Work out the finished part from the listing and answer in its coordinate system (mm). Face numbers are marked on the shaded views. A direction names the side the tool comes from. Round coordinates to 2 decimals unless told otherwise and drop trailing zeros. Loops run counter-clockwise (first coordinate to the right, second up) from the corner with the lowest first, then second, coordinate; pieces in that order, holes last. Notation, with made-up numbers: M -36.5,46.25 L -28.5,46.25 A8 ccw -28.5,52.25 Z; hole C 17.5,7.5 d4. An arc over 180 degrees is marked long. One line per item, written item: value.
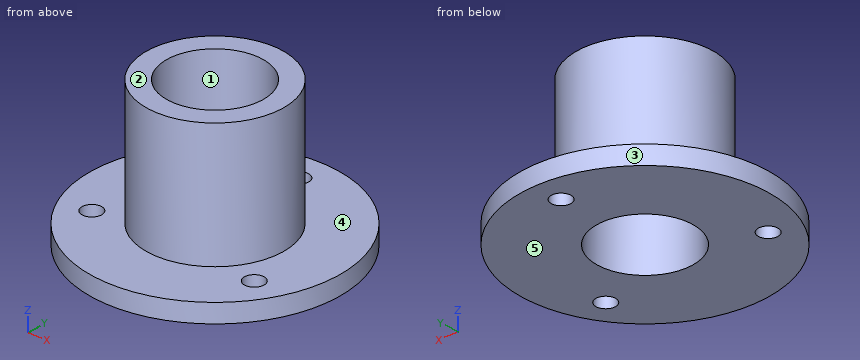
```python
from build123d import *

# Parameters (mm, degrees)
F0_R     = 11
F0_R_2   = 7.75
F1_DEPTH = 23
F0_R_3   = 20
F0_R_4   = 1.5875
F2_DEPTH = 3


with BuildPart() as f1:
    # F0 (on Top) → F1 (new body)
    with BuildSketch(Plane.XY):
        Circle(F0_R)
        Circle(F0_R_2, mode=Mode.SUBTRACT)
    extrude(amount=F1_DEPTH)

    # F0 (on Top) → F2 (join)
    with BuildSketch(Plane.XY):
        Circle(F0_R_3)
        with Locations((-13.282665, -7.66875)):
            Circle(F0_R_4, mode=Mode.SUBTRACT)
        with Locations((13.282665, -7.66875)):
            Circle(F0_R_4, mode=Mode.SUBTRACT)
        Circle(F0_R, mode=Mode.SUBTRACT)
        with Locations((0, 15.3375)):
            Circle(F0_R_4, mode=Mode.SUBTRACT)
    extrude(amount=F2_DEPTH)


solid = f1.part
```
1) Find section B-B (y = 0). Give the vertices of the cut face in (x, z).
Check values:
outline: M -20,0 L -7.75,0 L -7.75,23 L -11,23 L -11,3 L -20,3 Z; M 7.75,0 L 20,0 L 20,3 L 11,3 L 11,23 L 7.75,23 Z
2) Each of these flat-tipped pins is pushed along its axis until it touches: pin 1 (1.5 mm diameter, centred on y = 2, z = 7, fed in from +X); pin 2 (2 mm diameter, centred on x = 2, z = 6, fed in from +Y); pin 3 (4 mm diameter, centred on y = -10, z = 15.5, fed in from -X). Where does it stop, or does it pass through?
Check values:
pin 1: x = 10.93
pin 2: y = 10.95
pin 3: x = -7.55
3) For the marked faces 4 and 5, determine the directions among +Z, -Z, +X, -X, +Y, -Y from which every point of the face is accessible in a straight line to the end or side of a thin tool.
Check values:
face 4: +Z
face 5: -Z, +X, -X, +Y, -Y
4) Find section A-A (x = 0). Give the vertices of the cut face in (y, z) (3 decimals).
Check values:
outline: M -20,0 L -7.75,0 L -7.75,23 L -11,23 L -11,3 L -20,3 Z; M 7.75,0 L 13.75,0 L 13.75,3 L 11,3 L 11,23 L 7.75,23 Z; M 16.925,0 L 20,0 L 20,3 L 16.925,3 Z
5) Find section C-C (x = -6). Give the vertices of the cut face in (y, z), then the cut area to 3 significant figures.
Check values:
outline: M -19.08,0 L -4.91,0 L -4.91,23 L -9.22,23 L -9.22,3 L -19.08,3 Z; M 4.91,0 L 19.08,0 L 19.08,3 L 9.22,3 L 9.22,23 L 4.91,23 Z
area: 258 mm2
6) Find the intervals of material crossed by probe 1 along Y at (x, z) = (0, 1.35) (3 decimals); probe 2 along Y at (x, z) = (0, 15.5); probe 3 along Z at (x, y) = (-3, 14), in increasing order. Write a range as from..to.
Check values:
probe 1: -20..-7.75, 7.75..13.75, 16.925..20
probe 2: -11..-7.75, 7.75..11
probe 3: 0..3
7) The mould has two halves that part along Y. Classify the marked faces 1, 2 and 3: +Y half, -Y half, draft (parallel to the pull), parting line (faces both ways), or undercut.
Check values:
face 1: undercut
face 2: draft
face 3: parting line
8) Find section D-D (z = 2.5). Give the number of separate pieces and of enclosed holes in the cut face, then the cut area to 3 significant figures.
Check values:
separate pieces: 1
enclosed holes: 4
area: 1,040 mm2
